from build123d import *

# Parameters (mm, degrees)
SKETCH_5_R          = 1.5
CUT_EXTRUDE_2_DEPTH = 10
CUT_EXTRUDE_3_DEPTH = 10
SKETCH_7_W          = 6.5
SKETCH_7_H          = 3.804727479
CUT_EXTRUDE_4_DEPTH = 1.5


with BuildPart() as part:
    # Sketch 2 one side → Revolve 3 (revolve)
    with BuildSketch(Plane.XY):
        with BuildLine():
            Line((0, 0), (3.25, 0))
            Line((3.25, 0), (3.25, 3))
            Line((3.25, 3), (2.5, 3.733696482))
            Line((2.5, 3.733696482), (2.5, 12.207859217))
            ThreePointArc((2.5, 12.207859217), (2.525629935, 12.432810271), (2.601205954, 12.646230363))
            Line((2.601205954, 12.646230363), (5.392764278, 18.369773119))
            ThreePointArc((5.392764278, 18.369773119), (5.088288577, 24.179515585), (0, 27))
            Line((0, 27), (0, 0))
        make_face()
    revolve(axis=Axis((0, 35.781008953, 0), (0, -1, 0)))

    # Sketch 3 → Cut-Revolve 1 (revolve, cut)
    with BuildSketch(Plane(origin=(0, 0, 0), x_dir=(0, 0, -1), z_dir=(1, 0, 0))):
        with BuildLine():
            Line((0, 25), (0, 17))
            ThreePointArc((0, 17), (-4, 21), (0, 25))
        make_face()
    revolve(axis=Axis((0, 25, 0), (0, -1, 0)), mode=Mode.SUBTRACT)

    # Sketch 5 → Cut-Extrude 2 (cut)
    with BuildSketch(Plane.XZ):
        Circle(SKETCH_5_R)
    extrude(amount=-CUT_EXTRUDE_2_DEPTH, mode=Mode.SUBTRACT)

    # Sketch 6 → Cut-Extrude 3 (cut, symmetric)
    with BuildSketch(Plane(origin=(0, 0, 0), x_dir=(0, 0, -1), z_dir=(1, 0, 0))):
        Polygon((2.25, 28.432363899), (2.25, 13.369773119), (10.25, 5.369773119), (10.25, 28.432363899), align=None)
    cut_extrude_3 = extrude(amount=CUT_EXTRUDE_3_DEPTH, both=True, mode=Mode.SUBTRACT)

    # Mirror 1: Cut-Extrude 3 across plane
    add(cut_extrude_3.mirror(Plane.XY), mode=Mode.SUBTRACT)

    # Sketch 7 → Cut-Extrude 4 (cut, through all)
    with BuildSketch(Plane.XY.offset(2.75)):
        with Locations((0, 1.90236374)):
            Rectangle(SKETCH_7_W, SKETCH_7_H)
    cut_extrude_4 = extrude(amount=CUT_EXTRUDE_4_DEPTH, mode=Mode.SUBTRACT)

    # Mirror 2: Cut-Extrude 4 across plane
    add(cut_extrude_4.mirror(Plane.XY), mode=Mode.SUBTRACT)


solid = part.part
The listing builds one solid part. Answer for the finished solid, in the listing's coordinates (mm). A direction names the side the tool comes from. Coordinates: 2 decimals unless noted, no trailing zeros. Loops run counter-clockwise (first coordinate to the right, second up) from the corner with the lowest first, then second, coordinate; pieces in that order, holes last. Notation, with made-up numbers: M -18,86.25 L 1,86.25 A26 cw 1,104.25 Z; hole C 64,71.25 d6. An arc over 180 degrees is marked long. Answer in a Markdown table with one row per item.
1) Find the intervals of material crossed by probe 1 along Z at (x, y) = (0, 2.5); probe 2 along Y at (x, z) = (1.75, -2.15); probe 3 along Z at (x, y) = (0, 7.25), in increasing order.
Answers below:
| item | result |
|---|---|
| probe 1 | -2.75 to -1.5, 1.5 to 2.75 |
| probe 2 | 0 to 3.47, 13 to 18.12, 23.88 to 26.32 |
| probe 3 | -2.5 to -1.5, 1.5 to 2.5 |
2) Find section C-C (x = 0). Determine the outline of the cut face in (y, z), then the cut area to 3 significant figures.
Answers below:
| item | result |
|---|---|
| outline | M 0,-2.75 L 3.49,-2.75 L 3.73,-2.5 L 12.21,-2.5 A1 cw 12.65,-2.6 L 12.9,-2.72 L 13.37,-2.25 L 17.69,-2.25 A4 cw 17.69,2.25 L 13.37,2.25 L 12.9,2.72 L 12.65,2.6 A1 cw 12.21,2.5 L 3.73,2.5 L 3.49,2.75 L 0,2.75 L 0,1.5 L 10,1.5 L 10,-1.5 L 0,-1.5 Z; M 24.31,-2.25 L 26.56,-2.25 A6 ccw 26.56,2.25 L 24.31,2.25 A4 cw Z |
| area | 65.4 mm^2 |
3) Given pin 1 (1.5 mm diameter, centred on y = 13.5, z = 1.5, fed in from -X); pin 2 (5.5 mm diameter, centred on x = 0.5, y = 22, fed in from -Z); pin 3 (3 mm diameter, centred on x = -2, z = 2, fed in from +Y), each flat-ended and moving along its own axis, determine where each tip first touches the part or whether it passes through.
Answers below:
| item | result |
|---|---|
| pin 1 | x = -3.14 |
| pin 2 | z = -2.25 |
| pin 3 | y = 26.85 |
4) Find section A-A (y = 21.25). Determine the outline of the cut face in (x, z).
Answers below:
| item | result |
|---|---|
| outline | M -5.56,-2.25 L -3.3,-2.25 A3.99 cw -3.3,2.25 L -5.56,2.25 A5.99 ccw Z; M 3.3,-2.25 L 5.56,-2.25 A5.99 ccw 5.56,2.25 L 3.3,2.25 A3.99 cw Z |
5) Determine the mould class of faces 5 (the cylindrical face through (-1.5, 4.93, 0.07)), 6 (the flat face through (0, 10, 0)), 7 (the conical face through (2.85, 13.64, -1.18)), 8 (the flat face through (0, 17, 2.25)) for opening direction Z: released by +Z, released by -Z, zero draft, split by the parting line, or undercut.
Answers below:
| item | result |
|---|---|
| face 5 | undercut |
| face 6 | undercut |
| face 7 | split by the parting line |
| face 8 | released by +Z |
6) Find section B-B (z = 0). Determine the outline of the cut face in (x, y).
Answers below:
| item | result |
|---|---|
| outline | M -5.39,18.37 L -2.6,12.65 A1 cw -2.5,12.21 L -2.5,3.73 L -3.25,3 L -3.25,0 L -1.5,0 L -1.5,10 L 1.5,10 L 1.5,0 L 3.25,0 L 3.25,3 L 2.5,3.73 L 2.5,12.21 A1 cw 2.6,12.65 L 5.39,18.37 A6 ccw long Z; hole C 0,21 d8 |
7) Find section D-D (y = 6). Determine the outline of the cut face in (x, z), then the cut area to 3 significant figures.
Answers below:
| item | result |
|---|---|
| outline | C 0,0 d5; hole C 0,0 d3 |
| area | 12.6 mm^2 |
8) Which of the six approach directions +Z, -Z, +X, -X, +Y, -Y give full straight-line access (tool end or side, diameter ignored) to faces 1 (the cylindrical face through (3.25, 1.52, -0.05)), 2 (the cylindrical face through (-3.25, 1.52, 0.05)), 3 (the flat face through (0, 17, -2.25)), 4 (the cylindrical face through (-0.54, 8.03, -2.44))?
Answers below:
| item | result |
|---|---|
| face 1 | +X, -Y |
| face 2 | -X, -Y |
| face 3 | -Z, +X, -X, +Y |
| face 4 | none |
